from build123d import *

# Parameters (mm, degrees)
SKETCH_1_W          = 37
SKETCH_1_H          = 18.5
EXTRUDE_1_DEPTH     = 11
EXTRUDE_2_DEPTH     = 10
EXTRUDE_3_DEPTH     = 13.4
SKETCH_4_W          = 4.285372044
SKETCH_4_H          = 1.354621624
EXTRUDE_4_DEPTH     = 3
SKETCH_5_R          = 2
EXTRUDE_5_DEPTH     = 1
SKETCH_6_R          = 1.5
CUT_EXTRUDE_1_DEPTH = 20
SKETCH_8_R          = 2.75
EXTRUDE_6_DEPTH     = 9


with BuildPart() as part:
    # 스케치1 → 보스-돌출1 (new, symmetric)
    with BuildSketch(Plane.XY):
        Rectangle(SKETCH_1_W, SKETCH_1_H)
    extrude(amount=EXTRUDE_1_DEPTH, both=True)

    # 스케치2 → 보스-돌출2 (add)
    with BuildSketch(Plane.ZY.offset(18.5)):
        with BuildLine():
            Line((-6.225208394, -9.5), (6.225208394, -9.5))
            ThreePointArc((6.225208394, -9.5), (10.976552571, -1.148838505), (7.353316024, 7.75))
            Line((7.353316024, 7.75), (-7.353316024, 7.75))
            ThreePointArc((-7.353316024, 7.75), (-10.976552571, -1.148838505), (-6.225208394, -9.5))
        make_face()
    extrude(amount=EXTRUDE_2_DEPTH)

    # 스케치3 → 보스-돌출3 (add)
    with BuildSketch(Plane.ZY.offset(28.5)):
        with BuildLine():
            Line((-6.068131559, -9), (6.068131559, -9))
            ThreePointArc((6.068131559, -9), (10.476417681, -1.134328554), (7.159068059, 7.25))
            Line((7.159068059, 7.25), (-7.159068059, 7.25))
            ThreePointArc((-7.159068059, 7.25), (-10.476417681, -1.134328554), (-6.068131559, -9))
        make_face()
    extrude(amount=EXTRUDE_3_DEPTH)

    # 스케치4 → 보스-돌출4 (add)
    with BuildSketch(Plane(origin=(18.5, 0, 0), x_dir=(0, 0, -1), z_dir=(1, 0, 0))):
        Rectangle(SKETCH_4_W, SKETCH_4_H)
    extrude(amount=EXTRUDE_4_DEPTH)

    # 스케치5 → 보스-돌출5 (add)
    with BuildSketch(Plane(origin=(0, 9.25, 0), x_dir=(1, 0, 0), z_dir=(0, 1, 0))):
        with Locations((-2.729015684, 0)):
            Circle(SKETCH_5_R)
    extrude(amount=EXTRUDE_5_DEPTH)

    # 스케치6 → 컷-돌출1 (cut)
    with BuildSketch(Plane(origin=(0, 9.25, 0), x_dir=(1, 0, 0), z_dir=(0, 1, 0))):
        with Locations(Location((-13.3, 8.5, 0), (0, 0, 180))):
            Circle(SKETCH_6_R)
        with Locations(Location((-13.3, -8.5, 0), (0, 0, 180))):
            Circle(SKETCH_6_R)
    extrude(amount=-CUT_EXTRUDE_1_DEPTH, mode=Mode.SUBTRACT)

    # 스케치8 → 보스-돌출6 (add)
    with BuildSketch(Plane(origin=(0, 9.25, 0), x_dir=(1, 0, 0), z_dir=(0, 1, 0))):
        with Locations((7.5, 0)):
            Circle(SKETCH_8_R)
    extrude(amount=EXTRUDE_6_DEPTH)


solid = part.part
CAD build for the part. Positions are in the model's coordinates, mm. A direction names the side the tool comes from. Round coordinates to 2 decimals unless told otherwise and drop trailing zeros. Loops run counter-clockwise (first coordinate to the right, second up) from the corner with the lowest first, then second, coordinate; pieces in that order, holes last.
(1) Cut at B-B (z = 4.5). Give the cut face in (x, y).
(2) Which spindle directions (+Z, -Z, +X, -X, +Y, -Y) get a long thin tool onto all of the face, cutting with end or side? Do faces 1 (the flat face through (-18.5, 8, -1)), 2 (the flat face through (20, 0.677, 0)), 3 (the flat face through (0, -9.25, 0)), 4 (the cylindrical face through (10.04, 13.69, 1.05)). Say none if no direction does.
(3) Wall check: line 1 along Z through (x, y) = (-13.3, 0.75); line 2 along Y through (x, z) = (7, 7.25); line 3 along X through (y, z) = (4.5, 3.5). Give the ranges that are in metal, low to high.
(4) Drop flat-ended pins along their axis: pin 1 (11 mm diameter, centred on x = -3.5, z = 1.5, fed in from +Y); pin 2 (1.5 mm diameter, centred on y = -1.5, z = 2, fed in from +X); pin 3 (2.5 mm diameter, centred on x = -13.3, z = -8.5, fed in from -Y); pin 4 (4 mm diameter, centred on x = -38.5, z = -3, fed in from +Y). Give the stop position or say it passes through.
(5) Two-plate mould, pull along Z, no slides. Class faces 5 (the cylindrical face through (-35.106, -1.264, 10.467)), 6 (the flat face through (0, 9.25, 0)), 7 (the cylindrical face through (-14.686, 0.13, -9.075)): +Z half, -Z half, draft (parallel to the pull), parting line (faces both ways), or undercut.
(6) Cut at D-D (y = 4.75). Give the cut face in (x, z).
(7) Cut at A-A (x = -13.3). Give the cut face in (y, z), plus the area to 3 significant figures.
(8) Cut at C-C (z = 8.5). Give the cut face in (x, y), plus the area to 3 significant figures.
Findings below:
1. outline: (-41.9, -9) - (-28.5, -9) - (-28.5, -9.5) - (-18.5, -9.5) - (-18.5, -9.25) - (18.5, -9.25) - (18.5, 9.25) - (-18.5, 9.25) - (-18.5, 7.75) - (-28.5, 7.75) - (-28.5, 7.25) - (-41.9, 7.25) - close
2. face 1: -X, +Y
2. face 2: +Z, -Z, +X, +Y
2. face 3: +Z, -Z, +X, -Y
2. face 4: +Y
3. line 1: z = -11 to -10, -7 to 7, 10 to 11
3. line 2: y = -9.25 to 9.25
3. line 3: x = -41.9 to 18.5
4. pin 1: stops at y = 10.25
4. pin 2: stops at x = 18.5
4. pin 3: passes through
4. pin 4: stops at y = 7.25
5. face 5: +Z half
5. face 6: draft
5. face 7: undercut
6. outline: (-41.9, -9.13) - (-28.5, -9.13) - (-28.5, -9.7) - (-18.5, -9.7) - (-18.5, -11) - (18.5, -11) - (18.5, 11) - (-18.5, 11) - (-18.5, 9.7) - (-28.5, 9.7) - (-28.5, 9.13) - (-41.9, 9.13) - close; hole circle Ø3 at (-13.3, -8.5); hole circle Ø3 at (-13.3, 8.5)
7. outline: (-9.25, -11) - (9.25, -11) - (9.25, -10) - (-9.25, -10) - close; (-9.25, -7) - (9.25, -7) - (9.25, 7) - (-9.25, 7) - close; (-9.25, 10) - (9.25, 10) - (9.25, 11) - (-9.25, 11) - close
7. area: 296 mm2
8. outline: (-41.9, -6.6) - (-28.5, -6.6) - (-28.5, -7.41) - (-18.5, -7.41) - (-18.5, -9.25) - (-14.8, -9.25) - (-14.8, 9.25) - (-18.5, 9.25) - (-18.5, 6.55) - (-28.5, 6.55) - (-28.5, 5.73) - (-41.9, 5.73) - close; (-11.8, -9.25) - (18.5, -9.25) - (18.5, 9.25) - (-11.8, 9.25) - close
8. area: 934 mm2
